Verification items for the finished model (mm, model axes). A direction names the side the tool comes from. Round coordinates to 2 decimals unless told otherwise and drop trailing zeros. Order: outer loops, then holes, each group sorted by start corner. A loop starts at its lowest first (then second) coordinate and runs counter-clockwise, first axis right, second up. Notation, with made-up numbers: M 81.25,70 L 124.25,70 A7 ccw 124.25,75 Z; hole C 62,30.5 d5. An arc over 180 degrees is marked long. Write item = value, one per line. Start each with the question number.
from build123d import *

# Parameters (mm, degrees)
SKETCH1_R           = 110.49
BOSS_EXTRUDE1_DEPTH = 25.4
SKETCH2_R           = 101.6
CUT_EXTRUDE6_DEPTH  = 64.52
CUT_EXTRUDE7_DEPTH  = 64.52
SCALE1_SCALE        = 0.5


with BuildPart() as part:
    # Sketch1 → Boss-Extrude1 (new body)
    with BuildSketch(Plane(origin=(0, 0, 0), x_dir=(1, 0, 0), z_dir=(0, 1, 0))):
        Circle(SKETCH1_R)
    extrude(amount=BOSS_EXTRUDE1_DEPTH)

    # Sketch2 → Cut-Extrude6 (cut)
    with BuildSketch(Plane(origin=(0, 25.4, 0), x_dir=(1, 0, 0), z_dir=(0, 1, 0))):
        Circle(SKETCH2_R)
    extrude(amount=-CUT_EXTRUDE6_DEPTH, mode=Mode.SUBTRACT)

    # Sketch5 → Cut-Extrude7 (cut)
    with BuildSketch(Plane(origin=(0, 25.4, 0), x_dir=(1, 0, 0), z_dir=(0, 1, 0))):
        with BuildLine():
            Line((-46.233713441, -90.471010503), (-55.233336601, -85.275075655))
            Line((-55.233336601, -85.275075655), (-57.601465369, -88.931243691))
            ThreePointArc((-57.601465369, -88.931243691), (-105.956098512, -0.010262293), (-57.618691018, 88.920084135))
            Line((-57.618691018, 88.920084135), (-55.249854064, 85.264374893))
            Line((-55.249854064, 85.264374893), (-46.225266875, 90.475326484))
            Line((-46.225266875, 90.475326484), (-48.207174741, 94.354455224))
            ThreePointArc((-48.207174741, 94.354455224), (52.995520175, 91.750584513), (105.819002137, 5.388293237))
            Line((105.819002137, 5.388293237), (101.468539496, 5.166768105))
            Line((101.468539496, 5.166768105), (101.478542465, -4.966429217))
            Line((101.478542465, -4.966429217), (105.829433983, -5.179364822))
            ThreePointArc((105.829433983, -5.179364822), (53.084989634, -91.698848372), (-48.209389303, -94.353323737))
            Line((-48.209389303, -94.353323737), (-46.233713441, -90.471010503))
        make_face()
    extrude(amount=-CUT_EXTRUDE7_DEPTH, mode=Mode.SUBTRACT)


with BuildPart() as part_1:
    # Scale1: scaled about (-0.039482606, 12.7, -0.004547928)
    add(part.part.scale(SCALE1_SCALE).moved(Location((-0.019741303, 6.35, -0.002273964))))


solid = part_1.part
1) Release check for a two-part mould opening along Z. For faces 1 (the cylindrical face through (-25.451, 12.789, 43.974)), 2 (the cylindrical face through (51.01, 12.61, 21.16)), 3 (the cylindrical face through (27.16, 12.79, 45.47)), 4 (the flat face through (-25, 19.05, 45)) record: pulls with the +Z half, pulls with the -Z half, needs draft (parallel to the pull), parting line crosses it, or undercut.
2) Access from +Z, -Z, +X, -X, +Y, -Y to the whole of each face (thin tool, end or side, straight path). Record for faces 5 (the cylindrical face through (-52.993, 12.789, 0.742)), 6 (the flat face through (-25, 6.35, 45)).
3) Cross-section at C-C, the plane y = 11.75. Enter the section's corners in (x, z) (1 decimal), then the cut area to 3 significant figures.
4) Cross-section at A-A, the plane x = -5. Enter the section's corners in (y, z).
5) Cross-section at B-B, the plane z = -35.5. Enter the section's corners in (x, y).
6) Gauge pin test, flat ends, axial feed: P1, Ø5, axis at y = 17.5, z = -34, coming from the -X side; P2, Ø3, axis at x = 7.5, y = 11, coming from the +Z side; P3, Ø6, axis at y = 10.5, z = -34, coming from the -X side. Record the tip position at first contact, or that the pin passes through.
7) Scan lines: probe 1 along X at (y, z) = (8.5, -1); probe 2 along X at (y, z) = (16.5, 44); probe 3 along Z at (x, y) = (9.5, 10.5). Record each from-to range of solid material in increasing order.
Geometry results:
q1.face_1 = undercut
q1.face_2 = parting line crosses it
q1.face_3 = undercut
q1.face_4 = needs draft
q2.face_5 = +Y, -Y
q2.face_6 = +Z, -Z, +X, -X, -Y
q3.outline = C 0,0 d110.5; hole M -28.8,-44.5 L -27.6,-42.6 A50.8 ccw -23.1,-45.2 L -24.1,-47.2 A53 ccw 52.9,-2.7 L 50.7,-2.6 A50.8 ccw 50.7,2.5 L 52.9,2.6 A53 ccw -24.1,47.2 L -23.1,45.2 A50.8 ccw -27.6,42.6 L -28.8,44.5 A53 ccw Z
q3.area = 805 mm^2
q4.outline = M 6.35,-55.02 L 19.05,-55.02 L 19.05,-52.75 L 6.35,-52.75 Z; M 6.35,52.74 L 19.05,52.74 L 19.05,55.02 L 6.35,55.02 Z
q5.outline = M -42.35,6.35 L -39.35,6.35 L -39.35,19.05 L -42.35,19.05 Z; M 39.31,6.35 L 42.31,6.35 L 42.31,19.05 L 39.31,19.05 Z
q6.P1 = -45.41
q6.P2 = 54.91
q6.P3 = -45.75
q7.probe_1 = -55.26 to -52.99, 50.77 to 55.22
q7.probe_2 = -33.42 to -29.52, -28.52 to -25.41, 29.48 to 33.38
q7.probe_3 = -54.42 to -52.12, 52.11 to 54.42
